Autodesk Inventor part; units mm, degrees
ref_plane "YZ Plane" through (0, 0, 0) normal (1, 0, 0) x (0, 1, 0)
ref_plane "XZ Plane" through (0, 0, 0) normal (0, 1, 0) x (-1, 0, 0)
ref_plane "XY Plane" through (0, 0, 0) normal (0, 0, 1) x (1, 0, 0)
sketch "Sketch1" plane through (0, 0, 0) normal (0, 0, 1) x (1, 0, 0)
  line L0 (0, 0) -> (30, 0)
  line L1 (30, 0) -> (30, 17.3)
  line L2 (30, 17.3) -> (0, 17.3)
  line L3 (0, 17.3) -> (0, 0)
  dimension "d0" = 30
  dimension "d1" = 17.3
extrude "Extrusion1" add sketch "Sketch1" along normal blind 2.5
sketch "Sketch2" plane through (0, 0, 2.5) normal (0, 0, 1) x (1, 0, 0)
  line L0 (0, 17.3) -> (0, 0)
  line L1 (0, 0) -> (30, 0)
  point P0 (7, 8)
  dimension "d4" = 7
  dimension "d12" = 8
hole "Hole1" at (7, 8, 2.5) direction (0, 0, -1) diameter 7.2 end through all
sketch "Sketch3" plane through (0, 0, 2.5) normal (0, 0, 1) x (1, 0, 0)
  line L0 (30, 0) -> (30, 17.3)
  line L1 (30, 0) -> (18, 0)
  line L2 (18, 0) -> (18, -2.5)
  line L3 (18, -2.5) -> (30, -2.5)
  line L4 (30, -2.5) -> (30, 0)
  point P0 (0, 0)
  dimension "d13" = 2.5
  dimension "d14" = 12
extrude "Extrusion2" add sketch "Sketch3" against normal blind 14
sketch "Sketch4" plane through (18, 0, 0) normal (0, 1, 0) x (1, 0, 0)
  line L0 (3.25, 3) -> (8.75, 3)
  line L1 (8.75, 3) -> (8.75, 8.5)
  line L2 (8.75, 8.5) -> (3.25, 8.5)
  line L3 (3.25, 8.5) -> (3.25, 3)
  line L4 (0, 0) -> (0, 11.5)
  line L5 (0, 11.5) -> (12, 11.5)
  point P0 (-18, 0)
  point P1 (3.25, 5.75)
  point P2 (0, 5.75)
  point P3 (6, 8.5)
  point P4 (6, 11.5)
  dimension "d17" = 5.5
extrude "Extrusion3" [suppressed]
fillet "Fillet1" [suppressed]
fillet "Fillet2" [suppressed]
fillet "Fillet3" radius 1 1 edges at (24, 0, 0)
sketch "Sketch5" plane through (0, 0, 0) normal (0, 0, -1) x (-1, 0, 0)
  line L0 (-30, 17.3) -> (0, 17.3)
  line L1 (-30, 1) -> (-30, 17.3)
  line L2 (0, 17.3) -> (0, 0)
  line L3 (-30, -2.5) -> (-30, 17.3)
  line L4 (0, 14.8) -> (-30, 14.8)
  point P0 (0, 2)
  dimension "d26" = 2.5
extrude "Extrusion4" add sketch "Sketch5" along normal blind 14
chamfer "Chamfer2" distance 2 angle 45 6 edges at (0, 0, 1.25) (18, -1.25, -11.5) (0, 16.05, -14) (30, 16.05, -14) (15, 17.3, 2.5) (30, -1.25, -11.5)
fillet "Fillet4" radius 1 1 edges at (15, 14.8, 0)
sketch "Sketch6" plane through (0, 17.3, 0.5) normal (0, 1, 0) x (1, 0, 0)
  line L0 (29.5, 12.1) -> (0.5, 12.1)
  line L1 (0.5, 12.1) -> (0.5, 1.7)
  line L2 (0.5, 1.7) -> (29.5, 1.7)
  line L3 (29.5, 1.7) -> (29.5, 12.1)
  line L4 (0, 12.5) -> (0, 0)
  line L5 (30, 12.5) -> (30, 0)
  line L6 (2, 14.5) -> (28, 14.5)
  point P0 (0, 0.5)
  dimension "d33" = 10.4
  dimension "d34" = 0.5
  dimension "d36" = 0.5
  dimension "d37" = 2.4
emboss "Emboss1" sketch "Sketch6" operation cut depth 0.2 direction (0, -1, 0)
properties part number "GF1002 mount"
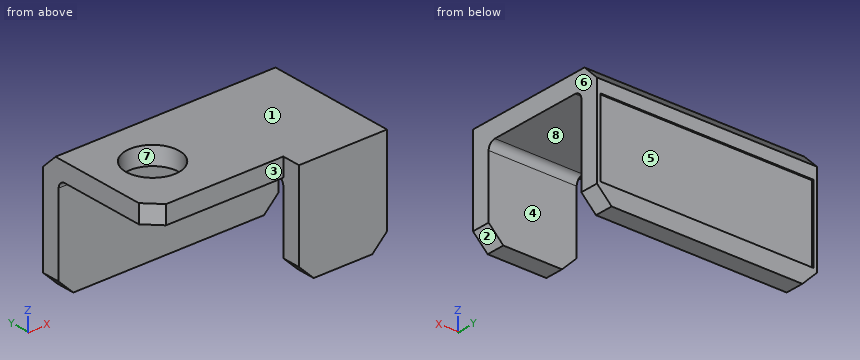
Read the model definition and answer for the solid it produces. Units are mm, in the model's axes. Face numbers are marked on the shaded views. A direction names the side the tool comes from. Give positions to 0.01 mm unless a question says otherwise; leave off trailing zeros. Write each loop counter-clockwise with the first axis right and the second up, starting at its lowest first coordinate (ties: lowest second). Pieces come first, ordered by that corner, then holes. Notation, with made-up numbers: M 80,85 L 119,85 A11 ccw 119,106 Z; hole C 16.25,25.5 d4. An arc over 180 degrees is marked long. Put each result on its own line as item: value. Start each with the question number.
1. The part is cut by section B-B, the plane z = -8.5. Give the vertices of the cut face in (x, y).
2. The part is cut by section D-D, the plane x = 12.25. Give the vertices of the cut face in (y, z), and give its area (3 significant figures).
3. For a pull along X with two mould halves and no side action, classify the marked faces 5, 6, 7 and 8 as released by +X, released by -X, zero draft, split by the parting line, or undercut.
4. The part is cut by section C-C, the plane y = 8. Give the vertices of the cut face in (x, z), and give its area (3 significant figures).
5. Which of the six approach directions +Z, -Z, +X, -X, +Y, -Y give full straight-line access (tool end or side, diameter ignored) to the marked faces 1, 2, 3 and 4?
6. The part is cut by section A-A, the plane x = 7. Give the vertices of the cut face in (y, z), and give its area (3 significant figures).
7. Consider line 1 along X through (y, z) = (8, 1.5); line 2 along Y through (x, z) = (12, -12); line 3 along Z through (x, y) = (19.5, 5.5). Determine where each line is inside the solid, lowest interval first.
8. Each of these flat-tipped pins is pushed along its axis until it touches: pin 1 Ø1.2 at (x, y) = (25, -1.5) entering from -Z; pin 2 Ø1.5 at (x, z) = (9.5, -3.5) entering from +Y; pin 3 Ø1 at (y, z) = (-1, -2.5) entering from -X. Where does it stop, or does it pass through?
Final values:
1. outline: M 0,14.8 L 30,14.8 L 30,17.3 L 29.5,17.3 L 29.5,17.1 L 0.5,17.1 L 0.5,17.3 L 0,17.3 Z; M 18,-2.5 L 30,-2.5 L 30,0 L 18,0 Z
2. outline: M 0,0 L 13.8,0 A1 cw 14.8,-1 L 14.8,-14 L 17.3,-14 L 17.3,-11.6 L 17.1,-11.6 L 17.1,-1.2 L 17.3,-1.2 L 17.3,0.5 L 15.3,2.5 L 0,2.5 Z
2. area: 74.4 mm²
3. face 5: undercut
3. face 6: released by +X
3. face 7: undercut
3. face 8: zero draft
4. outline: M 0,0 L 3.4,0 L 3.4,2.5 L 0,2.5 Z; M 10.6,0 L 30,0 L 30,2.5 L 10.6,2.5 Z
4. area: 57.0 mm²
5. face 1: +Z, +X, -X, +Y, -Y
5. face 2: -Z, +X, -Y
5. face 3: +Z, -Z, -X, -Y
5. face 4: -Z, +X, -X
6. outline: M 0,0 L 4.4,0 L 4.4,2.5 L 0,2.5 Z; M 11.6,0 L 13.8,0 A1 cw 14.8,-1 L 14.8,-14 L 17.3,-14 L 17.3,-11.6 L 17.1,-11.6 L 17.1,-1.2 L 17.3,-1.2 L 17.3,0.5 L 15.3,2.5 L 11.6,2.5 Z
6. area: 56.4 mm²
7. line 1: x = 0 to 3.4, 10.6 to 30
7. line 2: y = 14.8 to 17.3
7. line 3: z = 0 to 2.5
8. pin 1: stops at z = -11.5
8. pin 2: stops at y = 17.1
8. pin 3: stops at x = 18
